```python
from build123d import *

# Parameters (mm, degrees)
F0_W     = 50.8
F0_H     = 50.8
F1_DEPTH = 12.7
F2_W     = 50.8
F2_H     = 12.7
F3_DEPTH = 38.1
F5_DEPTH = 55.88


with BuildPart() as f1:
    # F0 (on Top) → F1 (new body)
    with BuildSketch(Plane.XY):
        with Locations((25.4, -25.4)):
            Rectangle(F0_W, F0_H)
    extrude(amount=F1_DEPTH)

    # F2 (on face) → F3 (join)
    with BuildSketch(Plane.XY.offset(12.7)):
        with Locations((25.4, -6.35)):
            Rectangle(F2_W, F2_H)
    extrude(amount=F3_DEPTH)

    # F4 (on face) → F5 (cut)
    with BuildSketch(Plane.XZ.offset(12.7)):
        with BuildLine():
            ThreePointArc((25.4, 38.1), (20.909872, 27.259872), (31.75, 31.75))
            ThreePointArc((31.75, 31.75), (29.890128, 36.240128), (25.4, 38.1))
        make_face()
    extrude(amount=-F5_DEPTH, mode=Mode.SUBTRACT)


solid = f1.part
```
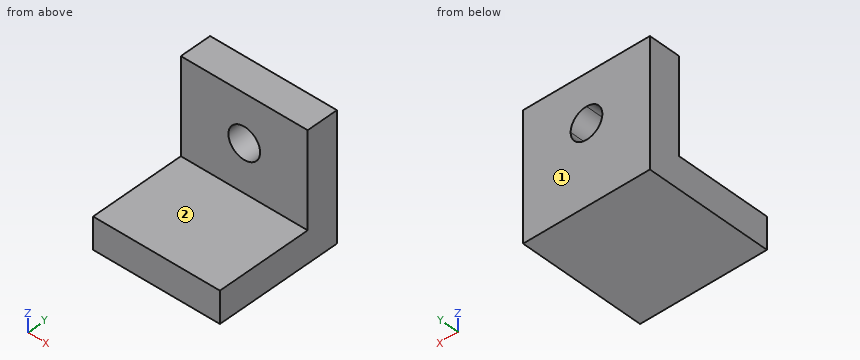
Part model, mm, in its own coordinate system. Face numbers are marked on the shaded views. A direction names the side the tool comes from. Give positions to 0.01 mm unless a question says otherwise; leave off trailing zeros. Order: outer loops, then holes, each group sorted by start corner. A loop starts at its lowest first (then second) coordinate and runs counter-clockwise, first axis right, second up. Notation, with made-up numbers: M -19.75,-19.75 L 22.25,-19.75 A23 ccw 22.25,14.25 Z; hole C 19,10.25 d2. An arc over 180 degrees is marked long. Use a Markdown table: item, result. Add a question column.
(1) Saw through at C-C, the plane z = 35. Give the cut face in (x, y), and give its area (3 significant figures).
(2) Drop flat-ended pins along their axis: P1, Ø3, axis at x = 29, z = 31.5, coming from the -Y side (3 decimals); P2, Ø19, axis at x = 18, z = 39, coming from the -Y side; P3, Ø2, axis at x = 12, y = -33, coming from the +Z side. Give the stop position or say it passes through.
(3) Saw through at B-B, the plane x = 29. Give the cut face in (y, z), and give its area (3 significant figures).
(4) 3-axis set-ups, long thin cutter, end or side, ignore diameter. For the marked faces 1 and 2: which of +Z, -Z, +X, -X, +Y, -Y reach the whole face in a straight line?
(5) Saw through at A-A, the plane y = -9.5. Give the cut face in (x, z).
(6) Probe line 1 along Z through (x, y) = (25, -8); line 2 along X through (y, z) = (-7.25, 31.75); line 3 along Y through (x, z) = (8.5, 44). List the from-to ranges inside material, lowest first. Write a range as [from, to].
(7) Saw through at D-D, the plane x = 38. Give the cut face in (y, z).
Answer key:
| question | item | result |
|---|---|---|
| 1 | outline | M 0,-12.7 L 19.94,-12.7 L 19.94,0 L 0,0 Z; M 30.86,-12.7 L 50.8,-12.7 L 50.8,0 L 30.86,0 Z |
| 1 | area | 507 mm^2 |
| 2 | P1 | through |
| 2 | P2 | y = -12.7 |
| 2 | P3 | z = 12.7 |
| 3 | outline | M -50.8,0 L 0,0 L 0,26.52 L -12.7,26.52 L -12.7,12.7 L -50.8,12.7 Z; M -12.7,36.98 L 0,36.98 L 0,50.8 L -12.7,50.8 Z |
| 3 | area | 996 mm^2 |
| 4 | face 1 | +Z, -Z, +X, -X, +Y |
| 4 | face 2 | +Z, +X, -X, -Y |
| 5 | outline | M 0,0 L 50.8,0 L 50.8,50.8 L 0,50.8 Z; hole C 25.4,31.75 d12.7 |
| 6 | line 1 | [0, 25.41], [38.09, 50.8] |
| 6 | line 2 | [0, 19.05], [31.75, 50.8] |
| 6 | line 3 | [-12.7, 0] |
| 7 | outline | M -50.8,0 L 0,0 L 0,50.8 L -12.7,50.8 L -12.7,12.7 L -50.8,12.7 Z |
